```python
from build123d import *

# Parameters (mm, degrees)
EXTRUDE_1_DEPTH = 5
EXTRUDE_2_DEPTH = 58
SKETCH_3_R      = 20
EXTRUDE_3_DEPTH = 5


with BuildPart() as part:
    # 草图1 → 凸台-拉伸1 (new body)
    with BuildSketch(Plane.XY):
        with BuildLine():
            Line((0, 0), (0, -190))
            ThreePointArc((0, -190), (134.350288425, -134.350288425), (190, 0))
            Line((190, 0), (0, 0))
        make_face()
    extrude(amount=EXTRUDE_1_DEPTH)

    # 草图2 → 凸台-拉伸2 (add)
    with BuildSketch(Plane(origin=(0, 0, 0), x_dir=(-1, 0, 0), z_dir=(0, 0, -1))):
        with BuildLine():
            Line((-5, -5), (-184.932420089, -5))
            ThreePointArc((-184.932420089, -5), (-130.81475452, -130.81475452), (-5, -184.932420089))
            Line((-5, -184.932420089), (-5, -5))
        make_face()
        with BuildLine():
            Line((-9.755273715, -10.014049165), (-9.755273715, -179.735457367))
            ThreePointArc((-9.755273715, -179.735457367), (-127.187558429, -127.370816834), (-179.721225289, -10.014049165))
            Line((-179.721225289, -10.014049165), (-9.755273715, -10.014049165))
        make_face(mode=Mode.SUBTRACT)
    extrude(amount=EXTRUDE_2_DEPTH)

    # 草图3 → 凸台-拉伸3 (add)
    with BuildSketch(Plane.XY.offset(5)):
        Circle(SKETCH_3_R)
    extrude(amount=-EXTRUDE_3_DEPTH)


solid = part.part
```
Geometry: final body of the model. Coordinates: model frame, mm. A direction names the side the tool comes from. Round coordinates to 2 decimals unless told otherwise and drop trailing zeros. Write each loop counter-clockwise with the first axis right and the second up, starting at its lowest first coordinate (ties: lowest second). Pieces come first, ordered by that corner, then holes.
Item 1: Section query B-B (x = 91). Return loops of the section in (y, z).
Item 2: Section query C-C (y = -62.5). Return loops of the section in (x, z), plus the area to 3 significant figures.
Item 3: Set-up query: faces 1 (the face through (94, -5, -29)), 2 (the face through (125.878, -128.665, -28.594)), 3 (the face through (132.196, -129.419, -28.594)), 4 (the face through (106, 0, 2)), 5 (the face through (0, -104, 2)). Return all of +Z, -Z, +X, -X, +Y, -Y with unobstructed straight access to the full face (end or side cutting, diameter ignored); none if empty.
Item 4: Section query A-A (z = -38). Return loops of the section in (x, y).
Item 5: Pin query (flat end, axial travel): P1, Ø3, axis at x = 51, z = -36.5, coming from the +Y side; P2, Ø4, axis at y = -72.5, z = -7, coming from the +X side; P3, Ø3, axis at x = 70.5, z = -41.5, coming from the -Y side. Return the tip coordinate at first contact, or that it passes through.
Item 6: Material intervals for L1, parallel to Z at x = 142, y = -25; L2, parallel to X at y = -130.5, z = -39; L3, parallel to X at y = -96.5, z = -3.5, sorted ascending.
Item 7: Mould query, pull axis X, two halves, no side actions, for faces 6 (the face through (75, -75, 0)), 7 (the face through (5, -96, -29)), 8 (the face through (132.865, -135.819, 2.465)), 9 (the face through (9.755, -94, -29)). Classes: +X half, -X half, draft (parallel to the pull), parting line (faces both ways), or undercut.
Completed:
1. outline: (-166.79, 0) - (-161.07, 0) - (-161.07, -58) - (-155.3, -58) - (-155.3, 0) - (-10.01, 0) - (-10.01, -58) - (-5, -58) - (-5, 0) - (0, 0) - (0, 5) - (-166.79, 5) - close
2. outline: (0, 0) - (5, 0) - (5, -58) - (9.76, -58) - (9.76, 0) - (168.8, 0) - (168.8, -58) - (174.12, -58) - (174.12, 0) - (179.43, 0) - (179.43, 5) - (0, 5) - close
2. area: 1,480 mm2
3. face 1: -Z, +X, -X, +Y
3. face 2: -Z
3. face 3: -Z, +X, -Y
3. face 4: +Z, -Z, +X, +Y
3. face 5: +Z, -Z, -X, -Y
4. outline: (5, -184.93) arc R185 ccw to (184.93, -5) - (5, -5) - close; hole (9.76, -179.74) arc R180 ccw to (179.72, -10.01) - (9.76, -10.01) - close
5. P1: stops at y = -5
5. P2: stops at x = 171.04
5. P3: stops at y = -171.65
6. L1: z = 0 to 5
6. L2: x = 5 to 9.76, 123.97 to 131.13
6. L3: x = 5 to 9.76, 151.95 to 157.84
7. face 6: undercut
7. face 7: -X half
7. face 8: +X half
7. face 9: undercut
